from build123d import *

# Parameters (mm, degrees)
SKETCH1_W           = 27.5
SKETCH1_H           = 27.8
SKETCH1_R           = 1.05
BOSS_EXTRUDE1_DEPTH = 1.2
SKETCH2_W           = 26.7
SKETCH2_H           = 19.25
BOSS_EXTRUDE2_DEPTH = 1.55
SKETCH3_W           = 17.75
SKETCH3_H           = 2.55
BOSS_EXTRUDE3_DEPTH = 2.35


with BuildPart() as part:
    # Sketch1 → Boss-Extrude1 (new body)
    with BuildSketch(Plane(origin=(0, 0, 0), x_dir=(1, 0, 0), z_dir=(0, 1, 0))):
        with Locations((-7.986995643, 4.078730041)):
            Rectangle(SKETCH1_W, SKETCH1_H)
        with Locations((-19.736995643, 15.678730041)):
            Circle(SKETCH1_R, mode=Mode.SUBTRACT)
        with Locations((3.763004357, 15.678730041)):
            Circle(SKETCH1_R, mode=Mode.SUBTRACT)
        with Locations((3.763004357, -7.521269959)):
            Circle(SKETCH1_R, mode=Mode.SUBTRACT)
        with Locations((-19.736995643, -7.521269959)):
            Circle(SKETCH1_R, mode=Mode.SUBTRACT)
    extrude(amount=BOSS_EXTRUDE1_DEPTH)

    # Sketch2 → Boss-Extrude2 (add)
    with BuildSketch(Plane(origin=(0, 1.2, 0), x_dir=(1, 0, 0), z_dir=(0, 1, 0))):
        with Locations((-7.986995643, 4.153730041)):
            Rectangle(SKETCH2_W, SKETCH2_H)
    extrude(amount=BOSS_EXTRUDE2_DEPTH)

    # Sketch3 → Boss-Extrude3 (add)
    with BuildSketch(Plane.XZ):
        with Locations((-7.256318238, -16.453730041)):
            Rectangle(SKETCH3_W, SKETCH3_H)
    extrude(amount=BOSS_EXTRUDE3_DEPTH)


solid = part.part
The listing builds one solid part. Answer for the finished solid, in the listing's coordinates (mm). A direction names the side the tool comes from. Give positions to 0.01 mm unless a question says otherwise; leave off trailing zeros. Loops run counter-clockwise (first coordinate to the right, second up) from the corner with the lowest first, then second, coordinate; pieces in that order, holes last. Notation, with made-up numbers: (77.25, -23) - (129.25, -23) arc R32 ccw to (129.25, 8) - close; hole circle Ø2 at (26.25, 25.25). An arc over 180 degrees is marked (long way). Use one line per item in the form item = value.
1. Which of the six approach directions +Z, -Z, +X, -X, +Y, -Y give full straight-line access (tool end or side, diameter ignored) to faces 5 (the face through (1.619, -1, -16)), 6 (the face through (-21.337, 2, -4)), 7 (the face through (-7, -1, -15.179)), 8 (the face through (-16.131, -1, -16))?
Calculated:
face_5 = +Z, -Z, +X, -Y
face_6 = +Z, -Z, -X, +Y
face_7 = +Z, +X, -X, -Y
face_8 = +Z, -Z, -X, -Y
2. Section B-B on z = -7 is taken. Give the vertices of the cut face in (x, y).
Calculated:
outline = (-21.74, 0) - (5.76, 0) - (5.76, 1.2) - (5.36, 1.2) - (5.36, 2.75) - (-21.34, 2.75) - (-21.34, 1.2) - (-21.74, 1.2) - close
3. The mould has two halves that part along Z. Classify faces 1 (the face through (2.93, 0.59, 8.16)), 2 (the face through (3.535, 0.592, -14.654)), 3 (the face through (-7, -1, -17.729)), 4 (the face through (-8, 2.75, -4)): pulls with the +Z half, pulls with the -Z half, needs draft (parallel to the pull), parting line crosses it, or undercut.
Calculated:
face_1 = undercut
face_2 = undercut
face_3 = pulls with the -Z half
face_4 = needs draft
4. Section A-A on x = 3.75 is taken. Give the vertices of the cut face in (y, z), then the cut area to 3 significant figures.
Calculated:
outline = (0, -17.98) - (1.2, -17.98) - (1.2, -16.73) - (0, -16.73) - close; (0, -14.63) - (1.2, -14.63) - (1.2, -13.78) - (2.75, -13.78) - (2.75, 5.47) - (1.2, 5.47) - (1.2, 6.47) - (0, 6.47) - close; (0, 8.57) - (1.2, 8.57) - (1.2, 9.82) - (0, 9.82) - close
area = 58.2 mm^2
5. Section C-C on x = -15 is taken. Give the vertices of the cut face in (y, z).
Calculated:
outline = (-2.35, -17.73) - (0, -17.73) - (0, -17.98) - (1.2, -17.98) - (1.2, -13.78) - (2.75, -13.78) - (2.75, 5.47) - (1.2, 5.47) - (1.2, 9.82) - (0, 9.82) - (0, -15.18) - (-2.35, -15.18) - close
6. Given pin 1 Ø1.3 at (x, z) = (3.76, -15.68) entering from +Y; pin 2 Ø12 at (x, z) = (-11.5, 1) entering from -Y; pin 3 Ø2.5 at (x, z) = (3.76, 7.52) entering from +Y; pin 4 Ø1.2 at (y, z) = (2, -4) entering from +X, each flat-ended and moving along its own axis, determine where each tip first touches the part or whether it passes through.
Calculated:
pin_1 = through
pin_2 = 0
pin_3 = 1.2
pin_4 = 5.36
7. Find the intervals of material crossed by line 1 along Y through (x, z) = (3.25, -1.75); line 2 along Z through (x, y) = (-4.5, 1.9); line 3 along Y through (x, z) = (-8.75, -14.5), in increasing order. Write a range as [from, to].
Calculated:
line_1 = [0, 2.75]
line_2 = [-13.78, 5.47]
line_3 = [0, 1.2]
8. Section D-D on y = 0.8 is taken. Give the vertices of the cut face in (x, z).
Calculated:
outline = (-21.74, -17.98) - (5.76, -17.98) - (5.76, 9.82) - (-21.74, 9.82) - close; hole circle Ø2.1 at (-19.74, -15.68); hole circle Ø2.1 at (-19.74, 7.52); hole circle Ø2.1 at (3.76, -15.68); hole circle Ø2.1 at (3.76, 7.52)
